```python
from build123d import *

# Parameters (mm, degrees)
F0_W = 9.525
F0_H = 1.524
F2_W = 5.715
F2_H = 19.05


# Not quite as in the source:
# - a fillet or chamfer that OpenCascade refuses, or shapes differently, is made with other operations: its cross-section is extruded or revolved along the edge and cut away or added


with BuildPart() as f1:
    # F0 (on Front) → F1 (revolve)
    with BuildSketch(Plane.XZ):
        with Locations((-4.7625, 0.762)):
            Rectangle(F0_W, F0_H)
    revolve(axis=Axis((0, 0, 0.762), (0, 0, 1)))

    # F2 (on Front) → F3 (revolve)
    with BuildSketch(Plane.XZ):
        with Locations((-2.8575, 9.525)):
            Rectangle(F2_W, F2_H)
    revolve(axis=Axis((0, 0, 9.525), (0, 0, 1)))

    # F4: fillet of radius 5.08 on 1 edges, made by hand

    # F4_s1 → F4_t2 (revolve)
    with BuildSketch(Plane.XZ):
        with BuildLine():
            ThreePointArc((-9.525, 1.524), (-6.7789073716, 3.3318368763), (-5.715, 6.4426888497))
            Line((-5.715, 6.4426888497), (-5.6134, 6.4426888497))
            Line((-5.6134, 6.4426888497), (-5.6134, 1.524))
            Line((-5.6134, 1.524), (-5.715, 1.4224))
            ThreePointArc((-5.715, 1.4224), (-7.62, 1.4224), (-9.4996, 1.425626223))
            Line((-9.4996, 1.425626223), (-9.525, 1.524))
        make_face()
    revolve(axis=Axis((0, 0, 1.524), (0, 0, -1)))


solid = f1.part
```
Verification items for the finished model (mm, model axes). A direction names the side the tool comes from. Give positions to 0.01 mm unless a question says otherwise; leave off trailing zeros. Loops run counter-clockwise (first coordinate to the right, second up) from the corner with the lowest first, then second, coordinate; pieces in that order, holes last.
1. Section check A-A, the plane x = 0. Enter the section's corners in (y, z) (3 decimals).
2. Section check D-D, the plane z = 5.25. Enter the section's corners in (x, y), then the cut area to 3 significant figures.
3. Set-up check for faces 1 (the flat face through (0, 0, 0)), 2 (the cylindrical face through (-5.45, -1.72, 12.83)): record each of +Z, -Z, +X, -X, +Y, -Y from which the full face is reachable in a straight line by a thin tool's end or side.
4. Go/stop test with flat-tipped pins: pin 1 Ø1 at (y, z) = (-0.5, 5) entering from +X; pin 2 Ø10 at (y, z) = (0.5, 7.5) entering from +X; pin 3 Ø8 at (x, z) = (-5, 12.5) entering from -Y; pin 4 Ø1.5 at (x, z) = (-6.5, 14.5) entering from -Y. Record where each tip stops, or that it passes through.
5. Thickness scan on line 1 (X direction, y = 0, z = 17.5) (3 decimals); line 2 (Z direction, x = 7.5, y = 0); line 3 (X direction, y = -0.75, z = 3.25). Record the ranges inside material, lowest first.
6. Section check C-C, the plane z = 11. Enter the section's corners in (x, y) (3 decimals), then the cut area to 3 significant figures.
Geometry says:
1. outline: (-9.525, 0) - (9.525, 0) - (9.525, 1.524) arc R5.08 cw to (5.715, 6.443) - (5.715, 19.05) - (-5.715, 19.05) - (-5.715, 6.443) arc R5.08 cw to (-9.525, 1.524) - close
2. outline: circle Ø11.71 at (0, 0)
2. area: 108 mm2
3. face 1: -Z, +X, -X, +Y, -Y
3. face 2: +Z
4. pin 1: stops at x = 6.08
4. pin 2: stops at x = 7.58
4. pin 3: stops at y = -5.63
4. pin 4: passes through
5. line 1: x = -5.715 to 5.715
5. line 2: z = 0 to 2.58
5. line 3: x = -6.8 to 6.8
6. outline: circle Ø11.43 at (0, 0)
6. area: 103 mm2
